Answer from the drawing. Dimensions are ordinates in mm from the lowest x, y and z of the part. Give positions to 0.01 mm unless a question says otherwise; leave off trailing zeros. Order: outer loops, then holes, each group sorted by start corner. A loop starts at its lowest first (then second) coordinate and runs counter-clockwise, first axis right, second up. Notation, with made-up numbers: M -5.75,18 L 37.25,18 A34 ccw 37.25,48 Z; hole C 37,6 d11. An arc over 180 degrees is marked long. One line per item, written item: value.
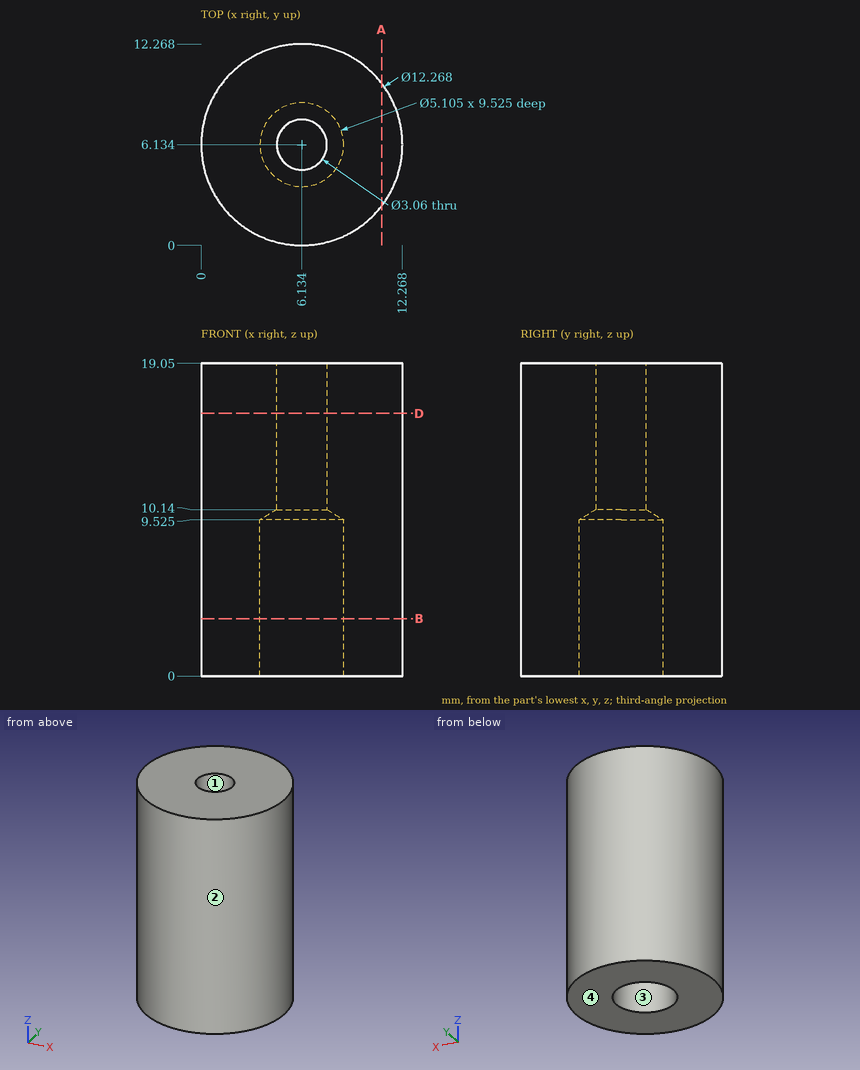
(1) Find the intervals of material crossed by probe 1 along Y at (x, z) = (6, 8.75) (1 decimal); probe 2 along X at (y, z) = (5, 8.75) (1 decimal), in increasing order. Write a range as from..to.
Findings:
probe 1: y = 0..3.6, 8.7..12.3
probe 2: x = 0.1..3.8, 8.4..12.2
(2) Section A-A, the plane x = 11 is taken. Give the vertices of the cut face in (y, z).
Findings:
outline: M 2.4,0 L 9.87,0 L 9.87,19.05 L 2.4,19.05 Z
(3) Section D-D, the plane z = 16 is taken. Give the vertices of the cut face in (x, y) (1 decimal), then the cut area to 3 significant figures.
Findings:
outline: C 6.1,6.1 d12.3; hole C 6.1,6.1 d3.1
area: 111 mm^2
(4) Given P1, Ø4, axis at x = 5, z = 4, coming from the -Y side; P2, Ø4.5, axis at x = 6.13, y = 6.13, coming from the -Z side; P3, Ø6, axis at y = 10, z = 8, coming from the -X side; P4, Ø6, axis at x = 10, z = 14, coming from the +Y side, each flat-ended and moving along its own axis, determine where each tip first touches the part or whether it passes through.
Findings:
P1: stops at y = 0
P2: stops at z = 9.7
P3: stops at x = 0.06
P4: stops at y = 12.21
(5) Section B-B, the plane z = 3.5 is taken. Give the vertices of the cut face in (x, y) (1 decimal).
Findings:
outline: C 6.1,6.1 d12.3; hole C 6.1,6.1 d5.1
(6) Determine the mould class of the marked faces 1, 2, 3 and 4 for opening direction Y: pulls with the +Y half, pulls with the -Y half, needs draft (parallel to the pull), parting line crosses it, or undercut.
Findings:
face 1: undercut
face 2: parting line crosses it
face 3: undercut
face 4: needs draft
